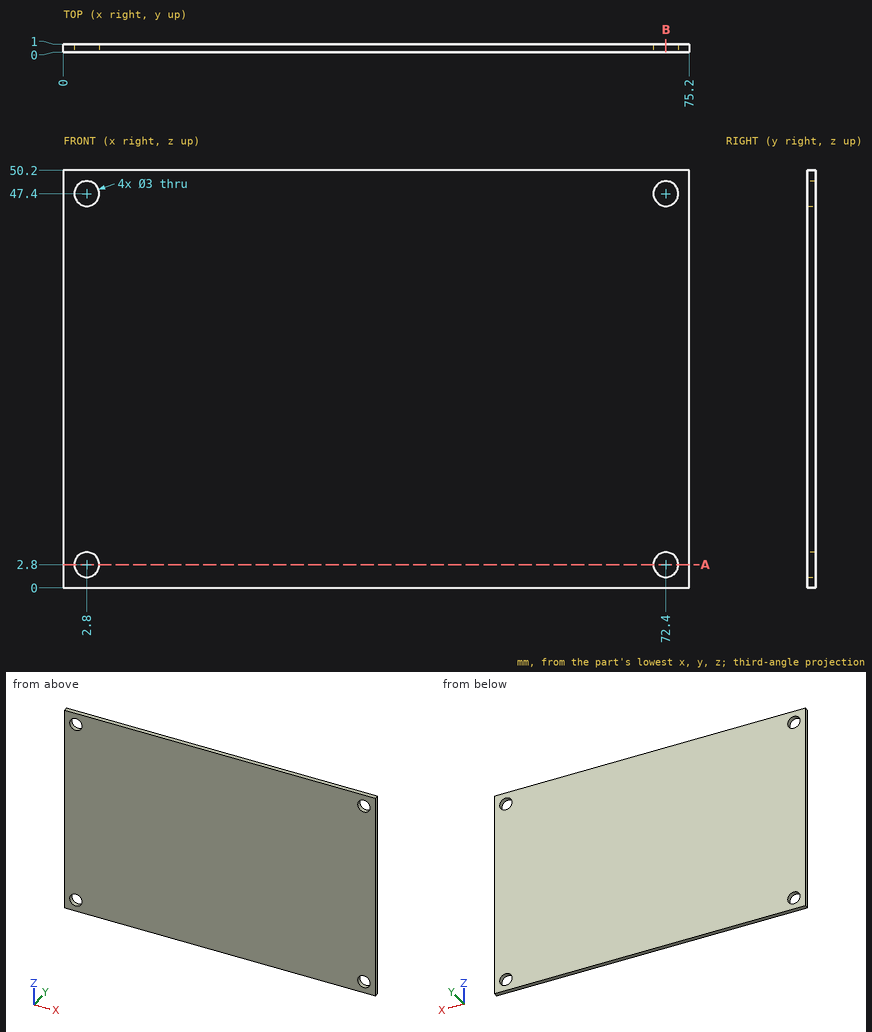
Input: dimensioned drawing with shaded views. Units: mm. Origin: part minimum x, y, z. Give positions to 0.01 mm unless a question says otherwise; leave off trailing zeros. Write each loop counter-clockwise with the first axis right and the second up, starting at its lowest first coordinate (ties: lowest second). Pieces come first, ordered by that corner, then holes.
Q1. First-contact query: P1, Ø2.5, axis at x = 72.4, z = 2.8, coming from the -Y side. Flat tip, straight axial feed; report the tip coordinate or a pass-through.
Q2. Section B-B, the plane x = 72.4. Output: boundary loops of the cut face in (y, z), plus the area to 3 significant figures.
Q3. Section A-A, the plane z = 2.8. Output: boundary loops of the cut face in (x, y), plus the area to 3 significant figures.
Q4. Material intervals for probe 1 along X at (y, z) = (0.2, 2.8); probe 2 along Z at (x, y) = (72.4, 0.25), sorted ascending.
Filled in:
1. P1: passes through
2. outline: (0, 0) - (1, 0) - (1, 1.3) - (0, 1.3) - close; (0, 4.3) - (1, 4.3) - (1, 45.9) - (0, 45.9) - close; (0, 48.9) - (1, 48.9) - (1, 50.2) - (0, 50.2) - close
2. area: 44.2 mm2
3. outline: (0, 0) - (1.3, 0) - (1.3, 1) - (0, 1) - close; (4.3, 0) - (70.9, 0) - (70.9, 1) - (4.3, 1) - close; (73.9, 0) - (75.2, 0) - (75.2, 1) - (73.9, 1) - close
3. area: 69.2 mm2
4. probe 1: x = 0 to 1.3, 4.3 to 70.9, 73.9 to 75.2
4. probe 2: z = 0 to 1.3, 4.3 to 45.9, 48.9 to 50.2
